```python
from build123d import *

# Parameters (mm, degrees)
F0_W     = 20
F0_H     = 10
F1_DEPTH = 25
F3_D     = 2.5
F3_DEPTH = 9.5
F3_TIP   = 0.7510757738
F4_D     = 3.3
F4_DEPTH = 10
F4_TIP   = 0.9914200214


with BuildPart() as f1:
    # F0 (on Top) → F1 (new body)
    with BuildSketch(Plane.XY):
        Rectangle(F0_W, F0_H)
    extrude(amount=-F1_DEPTH)

    # F3
    with Locations(Plane(origin=(0, 0, -25), x_dir=(1, 0, 0), z_dir=(0, 0, -1))):
        with Locations((-5, 0), (5, 0)):
            Hole(F3_D / 2, depth=F3_DEPTH)
            with Locations((0, 0, -(F3_DEPTH + F3_TIP / 2))):  # 118° drill point
                Cone(0, F3_D / 2, F3_TIP, mode=Mode.SUBTRACT)

    # F4
    with Locations(Plane.XY):
        with Locations((-5, 0), (5, 0)):
            Hole(F4_D / 2, depth=F4_DEPTH)
            with Locations((0, 0, -(F4_DEPTH + F4_TIP / 2))):  # 118° drill point
                Cone(0, F4_D / 2, F4_TIP, mode=Mode.SUBTRACT)


solid = f1.part
```
Verification items for the finished model (mm, model axes). A direction names the side the tool comes from. Coordinates: 2 decimals unless noted, no trailing zeros. Write each loop counter-clockwise with the first axis right and the second up, starting at its lowest first coordinate (ties: lowest second). Pieces come first, ordered by that corner, then holes. Notation, with made-up numbers: M 43.25,65.5 L 101.25,65.5 A37 ccw 101.25,104.5 Z; hole C 57,48 d3. An arc over 180 degrees is marked long. Answer as a JSON object with one key per item and string values. Group by question number.
(1) Tool access check on faces 1 (the face through (-10, 0, -12)), 2 (the face through (6.65, 0.07, -5.07)), 3 (the face through (6.25, -0.05, -20.18)). Record the directions out of +Z, -Z, +X, -X, +Y, -Y that give a thin tool (end or side, any length) a straight path to the whole face; none if there is none.
(2) Release check for a two-part mould opening along Y. For faces 4 (the face through (0, 5, -12)), 5 (the face through (-5.286, 0.013, -10.819)), 6 (the face through (0, -5, -12)), 7 (the face through (0, 0, -25)) record: +Y half, -Y half, draft (parallel to the pull), parting line (faces both ways), or undercut.
(3) Material ranges on line 1 (X direction, y = 0, z = -4.5); line 2 (Y direction, x = 5, z = -21.5); line 3 (Y direction, x = -5, z = -7.5), recorded low to high.
(4) Gauge pin test, flat ends, axial feed: pin 1 (2 mm diameter, centred on x = 5, y = 0, fed in from +Z); pin 2 (2 mm diameter, centred on x = -5, y = 0, fed in from -Z). Record the tip position at first contact, or that the pin passes through.
(5) Cross-section at B-B, the plane z = -16. Record the cut outline in (x, y), and give its area (3 significant figures).
(6) Cross-section at A-A, the plane z = -6. Record the cut outline in (x, y), and give its area (3 significant figures).
Reply:
{
 "1": {"face 1": "+Z, -Z, -X, +Y, -Y", "face 2": "+Z", "face 3": "-Z"},
 "2": {"face 4": "+Y half", "face 5": "undercut", "face 6": "-Y half", "face 7": "draft"},
 "3": {"line 1": "-10 to -6.65, -3.35 to 3.35, 6.65 to 10", "line 2": "-5 to -1.25, 1.25 to 5", "line 3": "-5 to -1.65, 1.65 to 5"},
 "4": {"pin 1": "z = -10.39", "pin 2": "z = -15.35"},
 "5": {"outline": "M -10,-5 L 10,-5 L 10,5 L -10,5 Z; hole C -5,0 d2.5; hole C 5,0 d2.5", "area": "190 mm²"},
 "6": {"outline": "M -10,-5 L 10,-5 L 10,5 L -10,5 Z; hole C -5,0 d3.3; hole C 5,0 d3.3", "area": "183 mm²"}
}
